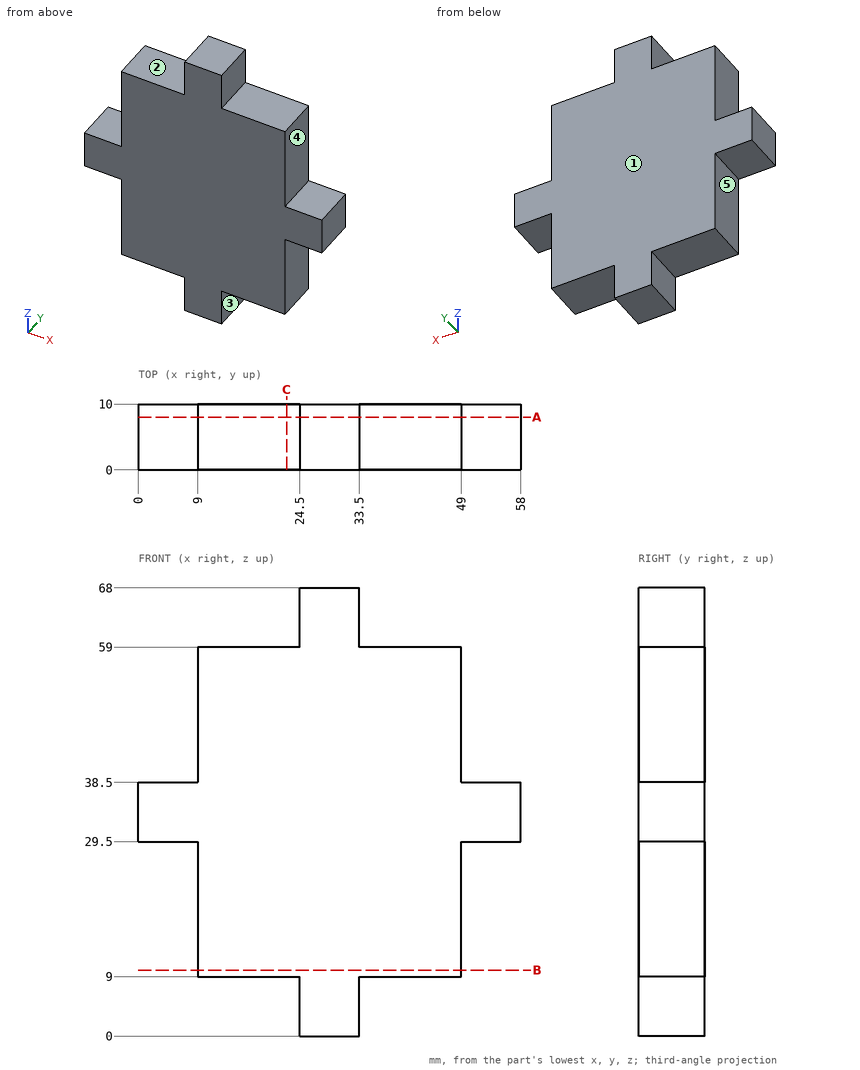
Here's the drawing with two shaded views (mm, measured from the low corner). I have some questions. A direction names the side the tool comes from. Give positions to 0.01 mm unless a question says otherwise; leave off trailing zeros. Order: outer loops, then holes, each group sorted by start corner. A loop starts at its lowest first (then second) coordinate and runs counter-clockwise, first axis right, second up.
Q1. If I drill on line 1 along X through (y, z) = (4, 23.5); line 2 along Z through (x, y) = (43, 0.5); line 3 along Z through (x, y) = (51, 6.25), over which ranges is the centre line in solid material (lowest first)?
Q2. Suppose I cut it at C-C, the plane x = 22.5. Write out the boundary of the cut face in (y, z), and give its area (3 significant figures).
Q3. I'm going to push flat-ended pins straight in: P1, Ø4.5, axis at x = 52, y = 5.5, coming from the +Z side; P2, Ø5, axis at y = 4.5, z = 45, coming from the +X side; P3, Ø5, axis at y = 5, z = 17, coming from the -X side. Where does each tip first touch, or does it pass through?
Q4. Suppose I cut it at A-A, the plane y = 8. Write out the boundary of the cut face in (x, z).
Q5. For the marked faces 1, 2, 3, 4 and 5, which set-ups out of +Z, -Z, +X, -X, +Y, -Y let a thin tool reach every point of the face, with its end or its side?
Q6. Suppose I cut it at B-B, the plane z = 10. Write out the boundary of the cut face in (x, y), and give its area (3 significant figures).
Solution:
1. line 1: x = 9 to 49
1. line 2: z = 9 to 59
1. line 3: z = 29.5 to 38.5
2. outline: (0, 9) - (10, 9) - (10, 59) - (0, 59) - close
2. area: 500 mm2
3. P1: stops at z = 38.5
3. P2: stops at x = 49
3. P3: stops at x = 9
4. outline: (0, 29.5) - (9, 29.5) - (9, 9) - (24.5, 9) - (24.5, 0) - (33.5, 0) - (33.5, 9) - (49, 9) - (49, 29.5) - (58, 29.5) - (58, 38.5) - (49, 38.5) - (49, 59) - (33.5, 59) - (33.5, 68) - (24.5, 68) - (24.5, 59) - (9, 59) - (9, 38.5) - (0, 38.5) - close
5. face 1: +Z, -Z, +X, -X, +Y
5. face 2: +Z, -X, +Y, -Y
5. face 3: -Z, +X, +Y, -Y
5. face 4: +Z, +X, +Y, -Y
5. face 5: -Z, -X, +Y, -Y
6. outline: (9, 0) - (49, 0) - (49, 10) - (9, 10) - close
6. area: 400 mm2
